Job drawing, mm, ordinate dimensions from the low corner. One solid piece. A direction names the side the tool comes from. Coordinates: 2 decimals unless noted, no trailing zeros. Loops run counter-clockwise (first coordinate to the right, second up) from the corner with the lowest first, then second, coordinate; pieces in that order, holes last. Notation, with made-up numbers: (18, 25) -> (77, 25) arc R27 cw to (77, 61) -> close; hole circle Ø4 at (-19.75, 4). An arc over 180 degrees is marked (long way). Answer as CSV lines item,"result". Start each with the question number.
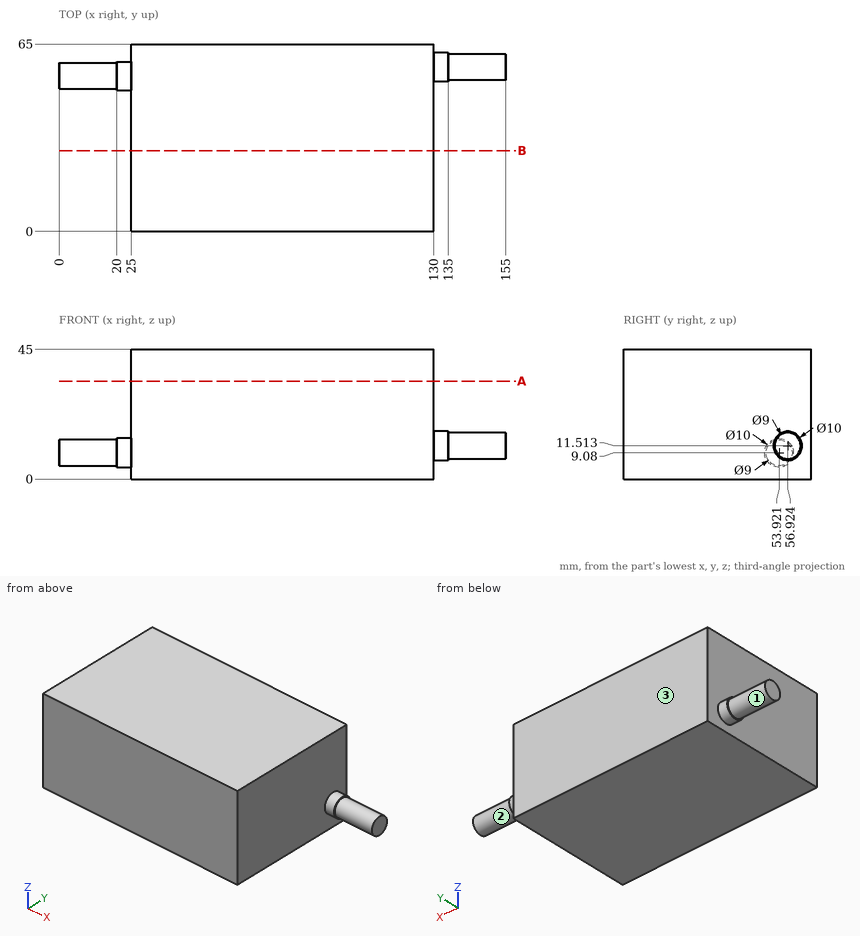
Q1. Probe probe 1 along X at (y, z) = (55, 24.5); probe 2 along X at (y, z) = (59, 9.5); probe 3 along Z at (x, y) = (146.5, 56). List the from-to ranges inside material, lowest first. Write a range as from..to.
Q2. Which spindle directions (+Z, -Z, +X, -X, +Y, -Y) get a long thin tool onto all of the face, cutting with end or side? Do the marked faces 1, 2 and 3. Say none if no direction does.
Q3. Saw through at B-B (y = 28). List the corners of the cut face in (x, z), and give its area (4 significant figures).
Q4. Pin check, flat tips, straight feed: pin 1 Ø8 at (y, z) = (55, 29.5) entering from -X; pin 2 Ø3 at (y, z) = (23.5, 34.5) entering from +X. Stop position of each tip, or through.
Q5. Saw through at A-A (z = 34). List the corners of the cut face in (x, y), and give its area (4 significant figures).
Ans:
1,probe 1,"x = 25..130"
1,probe 2,"x = 25..155"
1,probe 3,"z = 7.11..15.92"
2,face 1,"-X"
2,face 2,"+X"
2,face 3,"+Z, -Z, +X, -X, +Y"
3,outline,"(25, 0) -> (130, 0) -> (130, 45) -> (25, 45) -> close"
3,area,"4,725 mm²"
4,pin 1,"stops at x = 25"
4,pin 2,"stops at x = 130"
5,outline,"(25, 0) -> (130, 0) -> (130, 65) -> (25, 65) -> close"
5,area,"6,825 mm²"
